```python
from build123d import *

# Parameters (mm, degrees)
CROQUIS1_W              = 10
CROQUIS1_H              = 700
SALIENTE_EXTRUIR1_DEPTH = 200
CROQUIS2_R              = 10
CORTAR_EXTRUIR1_DEPTH   = 5


with BuildPart() as part:
    # Croquis1 → Saliente-Extruir1 (new body)
    with BuildSketch(Plane.XY):
        with Locations((5, 350)):
            Rectangle(CROQUIS1_W, CROQUIS1_H)
    extrude(amount=SALIENTE_EXTRUIR1_DEPTH)

    # Croquis2 → Cortar-Extruir1 (cut)
    with BuildSketch(Plane(origin=(10, 0, 0), x_dir=(0, 0, -1), z_dir=(1, 0, 0))):
        with Locations((-100, 110)):
            Circle(CROQUIS2_R)
        with Locations((-100, 230)):
            Circle(CROQUIS2_R)
        with Locations((-100, 350)):
            Circle(CROQUIS2_R)
        with Locations((-100, 470)):
            Circle(CROQUIS2_R)
        with Locations((-100, 590)):
            Circle(CROQUIS2_R)
    extrude(amount=-CORTAR_EXTRUIR1_DEPTH, mode=Mode.SUBTRACT)


solid = part.part
```
Can you work these out from the model? Positions are in its coordinate system, mm. A direction names the side the tool comes from. Round coordinates to 2 decimals unless told otherwise and drop trailing zeros. Loops run counter-clockwise (first coordinate to the right, second up) from the corner with the lowest first, then second, coordinate; pieces in that order, holes last. Notation, with made-up numbers: M 59,46 L 74,46 A17 ccw 74,50 Z; hole C 81.5,-26.5 d11. An arc over 180 degrees is marked long. Write item = value, one per line. Start each with the question number.
(1) Which directions (+Z, -Z, +X, -X, +Y, -Y) give clear straight access to the entire face, cutting with the end or side of a thin tool? Please do faces 1 (the face through (0, 345, 99)), 2 (the face through (7.535, 359.915, 101.302)).
(2) Suppose I cut it at B-B on z = 100. Write out the boundary of the cut face in (x, y).
(3) If we mould it in two halves opening along Z, with no side actions, what happens to faces 3 (the face through (10, 345, 76)), 4 (the face through (7.535, 599.915, 101.302)), 5 (the face through (5, 350, 100))? For each: released by +Z, released by -Z, zero draft, split by the parting line, or undercut.
(4) I need wall thicknesses on line 1 along Y through (x, z) = (8.3, 100); line 2 along Z through (x, y) = (6.5, 590). Which ranges of each line are inside material? Lowest first, please.
(5) Suppose I cut it at A-A on y = 230. Write out the boundary of the cut face in (x, z).
(6) I'm going to push a flat-ended pin straight in: P1, Ø6, axis at y = 346.5, z = 98, coming from the +X side. Where does the tip first touch, or does it pass through?
Answer block:
q1.face_1 = +Z, -Z, -X, +Y, -Y
q1.face_2 = +X
q2.outline = M 0,0 L 10,0 L 10,100 L 5,100 L 5,120 L 10,120 L 10,220 L 5,220 L 5,240 L 10,240 L 10,340 L 5,340 L 5,360 L 10,360 L 10,460 L 5,460 L 5,480 L 10,480 L 10,580 L 5,580 L 5,600 L 10,600 L 10,700 L 0,700 Z
q3.face_3 = zero draft
q3.face_4 = undercut
q3.face_5 = undercut
q4.line_1 = 0 to 100, 120 to 220, 240 to 340, 360 to 460, 480 to 580, 600 to 700
q4.line_2 = 0 to 90, 110 to 200
q5.outline = M 0,0 L 10,0 L 10,90 L 5,90 L 5,110 L 10,110 L 10,200 L 0,200 Z
q6.P1 = 5
